Autodesk Inventor part; units mm, degrees
ref_plane "YZ Plane" through (0, 0, 0) normal (1, 0, 0) x (0, 1, 0)
ref_plane "XZ Plane" through (0, 0, 0) normal (0, 1, 0) x (-1, 0, 0)
ref_plane "XY Plane" through (0, 0, 0) normal (0, 0, 1) x (1, 0, 0)
sketch "Sketch1" plane through (0, 0, 0) normal (0, 0, 1) x (1, 0, 0)
  line L0 (8.55, 7) -> (8.55, 13.2) construction
  line L1 (8.55, 13.2) -> (8.1046, 13.2) construction
  arc A0 (8.1046, 13.2) -> (8.1046, 7) centre (15.75, 10.1) ccw construction
  line L2 (8.1046, 7) -> (8.55, 7) construction
  line L3 (54.5, 18.2) -> (54.5, 16.6) construction
  line L4 (54.5, 16.6) -> (53.7436, 16.6) construction
  arc A1 (53.7436, 16.6) -> (53.7436, 13.6) centre (52, 15.1) ccw construction
  line L5 (53.7436, 13.6) -> (54.5, 13.6) construction
  line L6 (54.5, 13.6) -> (54.5, 6.6) construction
  line L7 (54.5, 6.6) -> (53.7436, 6.6) construction
  arc A2 (53.7436, 6.6) -> (53.7436, 3.6) centre (52, 5.1) ccw construction
  line L8 (53.7436, 3.6) -> (54.5, 3.6) construction
  line L9 (54.5, 3.6) -> (54.5, 2) construction
  arc A3 (52.5, 0) -> (54.5, 2) centre (52.5, 2) ccw construction
  line L10 (52.5, 0) -> (46.15, 0) construction
  arc A4 (46.15, 0) -> (47.65, 1.5) centre (46.15, 1.5) ccw construction
  line L11 (47.65, 18.7) -> (47.65, 1.5) construction
  arc A5 (47.65, 18.7) -> (46.15, 20.2) centre (46.15, 18.7) ccw construction
  line L12 (8.35, 20.2) -> (46.15, 20.2)
  arc A6 (8.35, 20.2) -> (6.85, 18.7) centre (8.35, 18.7) ccw construction
  line L13 (6.85, 1.5) -> (6.85, 18.7) construction
  arc A7 (6.85, 1.5) -> (8.35, 0) centre (8.35, 1.5) ccw construction
  line L14 (8.35, 0) -> (2, 0) construction
  arc A8 (0, 2) -> (2, 0) centre (2, 2) ccw construction
  line L15 (0, 2) -> (0, 3.6) construction
  line L16 (0, 3.6) -> (0.7564, 3.6) construction
  arc A9 (0.7564, 3.6) -> (0.7564, 6.6) centre (2.5, 5.1) ccw construction
  line L17 (0.7564, 6.6) -> (0, 6.6) construction
  line L18 (0, 6.6) -> (0, 13.6) construction
  line L19 (0, 13.6) -> (0.7564, 13.6) construction
  arc A10 (0.7564, 13.6) -> (0.7564, 16.6) centre (2.5, 15.1) ccw construction
  line L20 (0.7564, 16.6) -> (0, 16.6) construction
  line L21 (0, 16.6) -> (0, 18.2) construction
  arc A11 (2, 20.2) -> (0, 18.2) centre (2, 18.2) ccw construction
  line L22 (2, 20.2) -> (8.35, 20.2)
  arc A12 (54.5, 18.2) -> (52.5, 20.2) centre (52.5, 18.2) ccw construction
  line L23 (46.15, 20.2) -> (52.5, 20.2)
  line L24 (46.15, 0) -> (8.35, 0) construction
  line L25 (54.5, 0) -> (0, 0)
  line L26 (0, 0) -> (0, 20.2) construction
  line L27 (0, 20.2) -> (54.5, 20.2) construction
  line L28 (54.5, 20.2) -> (54.5, 0) construction
  line L29 (54.75, 20.45) -> (-0.25, 20.45)
  line L30 (-0.25, 20.45) -> (-0.25, -0.25)
  line L31 (-0.25, -0.25) -> (54.75, -0.25)
  line L32 (54.75, -0.25) -> (54.75, 20.45)
  line L33 (6.6, -0.25) -> (6.6, 20.45)
  line L34 (47.9, -0.25) -> (47.9, 20.45)
  circle A13 centre (2.5, 5.1) radius 1.9
  circle A14 centre (2.5, 15.1) radius 1.9
  circle A15 centre (52, 5.1) radius 1.9
  circle A16 centre (52, 15.1) radius 1.9
  point P0 (0, 0)
  point P1 (6.6, 20.2)
  point P2 (47.9, 20.2)
  point P3 (47.9, 0)
  point P4 (6.6, 0)
  dimension "d0" = 0
  dimension "d1" = 0
  dimension "d2" = 0.25
  dimension "d3" = 0
  dimension "d4" = 0
  dimension "d5" = 0.25
  dimension "d6" = 0.25
  dimension "d7" = 3.8
  dimension "d8" = 3.8
  dimension "d9" = 3.8
  dimension "d10" = 3.8
extrude "Extrusion1" add sketch "Sketch1" along normal blind 7 contours L22 L33 L29 L34 L23 L12 | L33 L31 L30 L29 | L34 L29 L32 L31 | L25 L34 L31 L33
ref_plane "Work Plane1" through (65.885, 15.7373, 10.7) normal (0, 0, -1) x (0.0023, 1, 0)
sketch "Sketch3" plane through (0, 0, 0) normal (0, 0, -1) x (-1, 0, 0)
  circle A0 centre (-51.2633, 10.1) radius 7.905 construction
  line L0 (10.9433, -15.3) -> (-77.9567, -15.3) construction
  line L1 (10.9433, 35.5) -> (10.9433, -15.3) construction
  line L2 (-77.9567, 35.5) -> (10.9433, 35.5) construction
  line L3 (-77.9567, -15.3) -> (-77.9567, 35.5) construction
  circle A1 centre (-15.75, 10.1) radius 7.905 construction
  line L4 (10.9433, -15.3) -> (-77.9567, -15.3)
  line L5 (-77.9567, -15.3) -> (-77.9567, 20.45)
  line L6 (-77.9567, 20.45) -> (10.9433, 20.45)
  line L7 (10.9433, 20.45) -> (10.9433, -15.3)
  line L8 (-54.75, 20.45) -> (0.25, 20.45)
  circle A2 centre (-52, 5.1) radius 1.9
  circle A3 centre (-52, 15.1) radius 1.9
  circle A4 centre (-2.5, 15.1) radius 1.9
  circle A5 centre (-2.5, 5.1) radius 1.9
  line L9 (-6.6, 0) -> (-6.6, 20.2)
  line L10 (-6.6, 20.2) -> (-47.9, 20.2)
  line L11 (-47.9, 20.2) -> (-47.9, 0)
  line L12 (-47.9, 0) -> (-6.6, 0)
  line L13 (-54.75, 20.45) -> (0.25, 20.45)
  line L14 (0.25, 20.45) -> (0.25, -0.25)
  line L15 (0.25, -0.25) -> (-54.75, -0.25)
  line L16 (-54.75, -0.25) -> (-54.75, 20.45)
  line L17 (10.9433, 20.45) -> (-77.9567, 20.45)
  line L18 (-77.9567, 20.45) -> (-77.9567, 22.45)
  line L19 (-77.9567, 22.45) -> (10.9433, 22.45)
  line L20 (10.9433, 22.45) -> (10.9433, 20.45)
  point P0 (0, 0)
  point P1 (0.25, 20.45)
  dimension "d16" = 0
  dimension "d19" = 2
extrude "Extrusion3" add sketch "Sketch3" against normal up to surface (7 mm away) contours L4 L5 L6 L16 L15 L14 L7 | L6 L18 L19 L20
sketch "Sketch4" plane through (0, 0, 7) normal (0, 0, 1) x (1, 0, 0)
  circle A0 centre (60.6, 3.5778) radius 1.9
  line L0 (-10.9433, 22.45) -> (77.9567, 22.45) construction
  line L1 (77.9567, 22.45) -> (77.9567, -15.3) construction
  line L2 (77.9567, -15.3) -> (-10.9433, -15.3) construction
  line L3 (-10.9433, -15.3) -> (-10.9433, 22.45) construction
  circle A1 centre (52, 5.1) radius 1.9 construction
  circle A2 centre (52, 15.1) radius 1.9 construction
  circle A3 centre (2.5, 15.1) radius 1.9 construction
  circle A4 centre (2.5, 5.1) radius 1.9 construction
  line L4 (6.6, 20.2) -> (6.6, 0) construction
  line L5 (6.6, 0) -> (47.9, 0) construction
  line L6 (47.9, 0) -> (47.9, 20.2) construction
  line L7 (47.9, 20.2) -> (6.6, 20.2) construction
  point P0 (0, 0)
  dimension "d20" = 3.8
  dimension "d21" = 18.8722
  dimension "d23" = 12.7
extrude "Extrusion4" cut sketch "Sketch4" against normal blind 6
properties part number "Top_Claw_Mount"
Can you work these out from the model? Positions are in its coordinate system, mm. A direction names the side the tool comes from. Give positions to 0.01 mm unless a question says otherwise; leave off trailing zeros. Order: outer loops, then holes, each group sorted by start corner. A loop starts at its lowest first (then second) coordinate and runs counter-clockwise, first axis right, second up. Notation, with made-up numbers: M -2,-27.5 L 14,-27.5 A26 ccw 14,6.5 Z; hole C -35,66 d11. An arc over 180 degrees is marked long. One line per question, with ' | ' between items.
Item 1: Please list where these lines run through material, in increasing order: L1, parallel to Y at x = 2.5, z = 3.5; L2, parallel to X at y = 16, z = 6.5; L3, parallel to Y at x = 25, z = 6.
Answer block:
L1: y = -15.3 to 3.2, 7 to 13.2, 17 to 22.45 | L2: x = -10.94 to 0.83, 4.17 to 6.6, 47.9 to 50.33, 53.67 to 77.96 | L3: y = -15.3 to 0, 20.2 to 22.45
Item 2: Suppose I cut it at C-C, the plane x = 31. Write out the boundary of the cut face in (y, z).
Answer block:
outline: M -15.3,0 L 0,0 L 0,7 L -15.3,7 Z; M 20.2,0 L 22.45,0 L 22.45,7 L 20.2,7 Z
Item 3: Suppose I cut it at A-A, the plane x = 52. Write out the boundary of the cut face in (y, z).
Answer block:
outline: M -15.3,0 L 3.2,0 L 3.2,7 L -15.3,7 Z; M 7,0 L 13.2,0 L 13.2,7 L 7,7 Z; M 17,0 L 22.45,0 L 22.45,7 L 17,7 Z
Item 4: For faces 1 (the face through (32.9, -0.4, 7)), 2 (the face through (62.355, 2.85, 4.042)), 3 (the face through (6.6, 10, 3)), which set-ups out of +Z, -Z, +X, -X, +Y, -Y let a thin tool reach every point of the face, with its end or its side?
Answer block:
face 1: +Z, +X, -X, +Y, -Y | face 2: +Z | face 3: +Z, -Z
Item 5: Suppose I cut it at B-B, the plane y = 15.1. Write out the boundary of the cut face in (x, z).
Answer block:
outline: M -10.94,0 L 0.6,0 L 0.6,7 L -10.94,7 Z; M 4.4,0 L 6.6,0 L 6.6,7 L 4.4,7 Z; M 47.9,0 L 50.1,0 L 50.1,7 L 47.9,7 Z; M 53.9,0 L 77.96,0 L 77.96,7 L 53.9,7 Z
Item 6: We'd pull the mould along Y, two halves only. Please class faces 4 (the face through (32.9, -0.4, 0)), 5 (the face through (34, 22.45, 3)), 6 (the face through (53.755, 5.828, 3.451)): released by +Y, released by -Y, zero draft, split by the parting line, or undercut.
Answer block:
face 4: zero draft | face 5: released by +Y | face 6: undercut
Item 7: Suppose I cut it at D-D, the plane z = 3.5. Write out the boundary of the cut face in (x, y), then the cut area to 3 significant figures.
Answer block:
outline: M -10.94,-15.3 L 77.96,-15.3 L 77.96,22.45 L -10.94,22.45 Z; hole C 2.5,5.1 d3.8; hole C 2.5,15.1 d3.8; hole M 6.6,0 L 47.9,0 L 47.9,20.2 L 6.6,20.2 Z; hole C 52,5.1 d3.8; hole C 52,15.1 d3.8; hole C 60.6,3.58 d3.8 | area: 2,470 mm2
